```python
from build123d import *

# Parameters (mm, degrees)
EXTRUDE_1_DEPTH       = 4
HOLE_WIZARD_5_0_5_1_D = 5
SKETCH_4_R            = 11.330923122
EXTRUDE_2_DEPTH       = 4.5
SKETCH_5_R            = 9.73271474
CUT_EXTRUDE_1_DEPTH   = 4.5
SKETCH_6_R            = 6
EXTRUDE_3_DEPTH       = 9
SKETCH_7_R            = 4
CUT_EXTRUDE_2_DEPTH   = 47.064049502


with BuildPart() as part:
    # 草图1 → 凸台-拉伸1 (new body)
    with BuildSketch(Plane.XY):
        with BuildLine():
            Line((-3.679866613, 4.367396682), (10.641275218, 10.64119661))
            ThreePointArc((10.641275218, 10.64119661), (18.25, 13.081580872), (25.858724782, 10.64119661))
            Line((25.858724782, 10.64119661), (40.179866613, 4.367396682))
            ThreePointArc((40.179866613, 4.367396682), (42.21100447, 0), (40.179866613, -4.367396682))
            Line((40.179866613, -4.367396682), (25.858724782, -10.64119661))
            ThreePointArc((25.858724782, -10.64119661), (18.25, -13.081580872), (10.641275218, -10.64119661))
            Line((10.641275218, -10.64119661), (-3.679866613, -4.367396682))
            ThreePointArc((-3.679866613, -4.367396682), (-5.71100447, 0), (-3.679866613, 4.367396682))
        make_face()
    extrude(amount=EXTRUDE_1_DEPTH)

    # Ø5.0 (5) 直径孔1 (through all)
    with Locations(Plane.XY.offset(4)):
        with Locations((0, 0), (36.5, 0)):
            Hole(HOLE_WIZARD_5_0_5_1_D / 2)

    # 草图4 → 凸台-拉伸2 (add)
    with BuildSketch(Plane.XY.offset(4)):
        with Locations((17.959725488, 0)):
            Circle(SKETCH_4_R)
    extrude(amount=EXTRUDE_2_DEPTH)

    # 草图5 → 切除-拉伸1 (cut)
    with BuildSketch(Plane.XY.offset(8.5)):
        with Locations((17.959725488, 0)):
            Circle(SKETCH_5_R)
    extrude(amount=-CUT_EXTRUDE_1_DEPTH, mode=Mode.SUBTRACT)

    # 草图6 → 凸台-拉伸3 (add)
    with BuildSketch(Plane.XY.offset(4)):
        with Locations((17.959725488, 0)):
            Circle(SKETCH_6_R)
    extrude(amount=EXTRUDE_3_DEPTH)

    # 草图7 → 切除-拉伸2 (cut, through all)
    with BuildSketch(Plane.XY.offset(13)):
        with Locations((17.959725488, 0)):
            Circle(SKETCH_7_R)
    extrude(amount=-CUT_EXTRUDE_2_DEPTH, mode=Mode.SUBTRACT)


solid = part.part
```
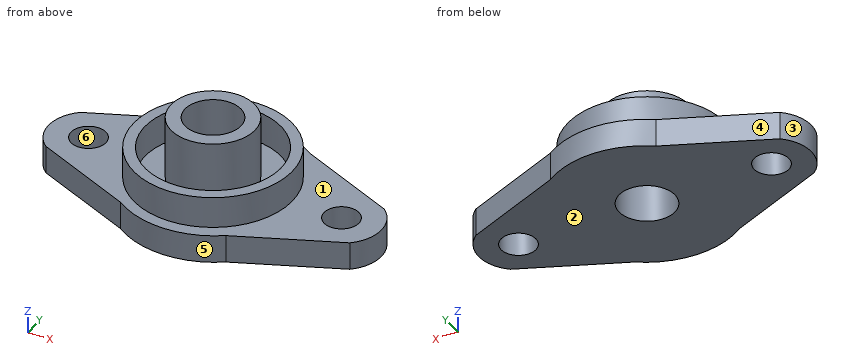
Check sheet for the modelled part. Datum: model origin and axes. Units: mm. Face numbers are marked on the shaded views. A direction names the side the tool comes from. Round coordinates to 2 decimals unless told otherwise and drop trailing zeros. Write each loop counter-clockwise with the first axis right and the second up, starting at its lowest first coordinate (ties: lowest second). Pieces come first, ordered by that corner, then holes. Notation, with made-up numbers: M 18,11 L 26,11 A17 cw 26,20 Z; hole C -25.5,-30 d10. An arc over 180 degrees is marked long. Write item = value, one per line. Start each with the question number.
1. Section check B-B, the plane y = 0. Record the cut outline in (x, z), then the cut area to 3 significant figures.
2. Section check A-A, the plane z = 2.75. Record the cut outline in (x, y).
3. Scan lines: line 1 (Y direction, x = 13, z = 6.75); line 2 (Y direction, x = 15, z = 7.5); line 3 (Y direction, x = 23, z = 4.5). Record each from-to range of solid material in increasing order. Write a range as [from, to].
4. Release check for a two-part mould opening along Y. For the marked faces 3, 4, 5 and 6 record: pulls with the +Y half, pulls with the -Y half, needs draft (parallel to the pull), parting line crosses it, or undercut.
5. Tool access check on the marked faces 1 and 2. Record the directions out of +Z, -Z, +X, -X, +Y, -Y that give a thin tool (end or side, any length) a straight path to the whole face; none if there is none.
6. Section check C-C, the plane z = 7. Record the cut outline in (x, y), then the cut area to 3 significant figures.
7. Gauge pin test, flat ends, axial feed: pin 1 (3 mm diameter, centred on x = -0.5, z = 2.5, fed in from +Y); pin 2 (3 mm diameter, centred on y = 4, z = 11, fed in from +X); pin 3 (6 mm diameter, centred on x = 33.5, y = -9, fed in from +Z). Record the tip position at first contact, or that the pin passes through.
8. Section check D-D, the plane x = 0. Record the cut outline in (y, z).
Results found:
q1.outline = M -5.71,0 L -2.5,0 L -2.5,4 L -5.71,4 Z; M 2.5,0 L 13.96,0 L 13.96,13 L 11.96,13 L 11.96,4 L 8.23,4 L 8.23,8.5 L 6.63,8.5 L 6.63,4 L 2.5,4 Z; M 21.96,0 L 34,0 L 34,4 L 29.29,4 L 29.29,8.5 L 27.69,8.5 L 27.69,4 L 23.96,4 L 23.96,13 L 21.96,13 Z; M 39,0 L 42.21,0 L 42.21,4 L 39,4 Z
q1.area = 170 mm^2
q2.outline = M -3.68,-4.37 L 10.64,-10.64 A13.08 ccw 25.86,-10.64 L 40.18,-4.37 A5.71 ccw 40.18,4.37 L 25.86,10.64 A13.08 ccw 10.64,10.64 L -3.68,4.37 A5.71 ccw Z; hole C 0,0 d5; hole C 17.96,0 d8; hole C 36.5,0 d5
q3.line_1 = [-10.19, -8.37], [-3.38, 3.38], [8.37, 10.19]
q3.line_2 = [-10.94, -9.27], [-5.22, -2.69], [2.69, 5.22], [9.27, 10.94]
q3.line_3 = [-10.15, -8.33], [-3.26, 3.26], [8.33, 10.15]
q4.face_3 = parting line crosses it
q4.face_4 = pulls with the +Y half
q4.face_5 = pulls with the -Y half
q4.face_6 = undercut
q5.face_1 = +Z
q5.face_2 = -Z, +X, -X, +Y, -Y
q6.outline = C 17.96,0 d22.66; C 17.96,0 d12; hole C 17.96,0 d19.47; hole C 17.96,0 d8
q6.area = 169 mm^2
q7.pin_1 = 6.42
q7.pin_2 = 23.41
q7.pin_3 = 4
q8.outline = M -5.98,0 L -2.5,0 L -2.5,4 L -5.98,4 Z; M 2.5,0 L 5.98,0 L 5.98,4 L 2.5,4 Z
